Can you work these out from the model? Positions are in its coordinate system, mm. Face numbers are marked on the shaded views. A direction names the side the tool comes from. Round coordinates to 2 decimals unless told otherwise and drop trailing zeros. Loops run counter-clockwise (first coordinate to the right, second up) from the corner with the lowest first, then second, coordinate; pieces in that order, holes last. Notation, with made-up numbers: M -36.5,-20 L 5.5,-20 A11 cw 5.5,0 Z; hole C -33,4.5 d5. An arc over 180 degrees is marked long. Answer as CSV lines item,"result".
from build123d import *

# Parameters (mm, degrees)
SKETCH_1_W          = 50
SKETCH_1_H          = 25
EXTRUDE_1_DEPTH     = 2
SKETCH_2_W          = 15.416574513
SKETCH_2_H          = 15.10736158
EXTRUDE_2_DEPTH     = 16.5
SKETCH_2_6_W        = 4.64276656
SKETCH_2_6_H        = 12.070908618
SKETCH_2_6_W_2      = 4.657076635
SKETCH_2_6_H_2      = 15.10736158
EXTRUDE_3_DEPTH     = 8
SKETCH_3_R          = 1.5
CUT_EXTRUDE_1_DEPTH = 33.457664734
FILLET_1_R          = 2


with BuildPart() as part:
    # Sketch 1 → Extrude 1 (new body)
    with BuildSketch(Plane(origin=(0, 0, 0), x_dir=(1, 0, 0), z_dir=(0, 1, 0))):
        Rectangle(SKETCH_1_W, SKETCH_1_H)
    extrude(amount=EXTRUDE_1_DEPTH)

    # Sketch 2 → Extrude 2 (add)
    with BuildSketch(Plane(origin=(0, 2, 0), x_dir=(1, 0, 0), z_dir=(0, 1, 0))):
        with Locations((6.307789338, 0)):
            Rectangle(SKETCH_2_W, SKETCH_2_H)
    extrude(amount=EXTRUDE_2_DEPTH)

    # Sketch 2_6 → Extrude 3 (add)
    with BuildSketch(Plane(origin=(0, 2, 0), x_dir=(1, 0, 0), z_dir=(0, 1, 0))):
        with Locations((-21.10123104, 1.518226481)):
            Rectangle(SKETCH_2_6_W, SKETCH_2_6_H)
        with Locations((21.418251887, 0)):
            Rectangle(SKETCH_2_6_W_2, SKETCH_2_6_H_2)
    extrude(amount=EXTRUDE_3_DEPTH)

    # Sketch 3 → Cut-Extrude 1 (cut, through all)
    with BuildSketch(Plane(origin=(0, 2, 0), x_dir=(1, 0, 0), z_dir=(0, 1, 0))):
        with Locations(Location((-22.25, 10.25, 0), (0, 0, 270))):
            Circle(SKETCH_3_R)
        with Locations(Location((22.25, 10.25, 0), (0, 0, 90))):
            Circle(SKETCH_3_R)
        with Locations(Location((22.25, -10.25, 0), (0, 0, 270))):
            Circle(SKETCH_3_R)
        with Locations(Location((-22.25, -10.25, 0), (0, 0, 90))):
            Circle(SKETCH_3_R)
    extrude(amount=-CUT_EXTRUDE_1_DEPTH, mode=Mode.SUBTRACT)

    # Fillet 1
    fillet_1_edges = [part.edges().sort_by_distance(p)[0] for p in [
        (25, 1, 12.5),
        (-25, 1, 12.5),
        (-25, 1, -12.5),
        (25, 1, -12.5),
    ]]
    fillet(fillet_1_edges, radius=FILLET_1_R)


solid = part.part
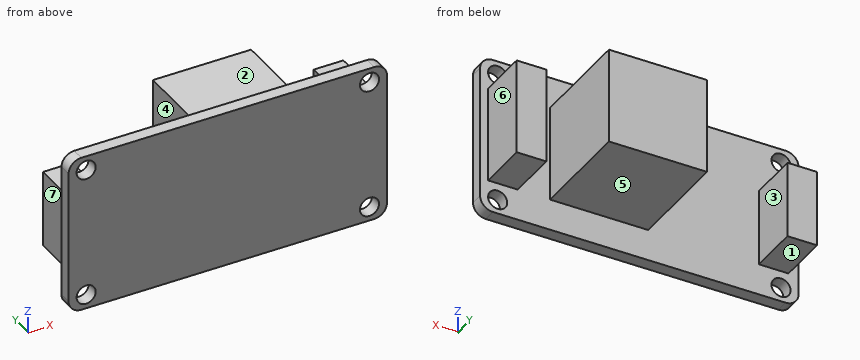
Item 1: If we section it at B-B on x = 22.25: Write out the boundary of the cut face in (y, z).
Output:
outline,"M 0,-12.5 L 2,-12.5 L 2,-11.75 L 0,-11.75 Z; M 0,-8.75 L 2,-8.75 L 2,-7.55 L 10,-7.55 L 10,7.55 L 2,7.55 L 2,8.75 L 0,8.75 Z; M 0,11.75 L 2,11.75 L 2,12.5 L 0,12.5 Z"
Item 2: If I drill on line 1 along X through (y, z) = (0.5, -10.25); line 2 along X through (y, z) = (8.25, -6.25); line 3 along X through (y, z) = (4.75, 5.5), over which ranges is the centre line in solid material (lowest first)? Write a range as from..to.
Output:
line 1,"x = -25..-23.75, -20.75..20.75, 23.75..25"
line 2,"x = -23.42..-18.78, -1.4..14.02, 19.09..23.75"
line 3,"x = -1.4..14.02, 19.09..23.75"
Item 3: If we section it at C-C on x = 0: Write out the boundary of the cut face in (y, z).
Output:
outline,"M 0,-12.5 L 2,-12.5 L 2,-7.55 L 18.5,-7.55 L 18.5,7.55 L 2,7.55 L 2,12.5 L 0,12.5 Z"
Item 4: We'd pull the mould along Z, two halves only. Please class the marked faces 1, 2 and 3: released by +Z, released by -Z, zero draft, split by the parting line, or undercut.
Output:
face 1,"released by -Z"
face 2,"released by +Z"
face 3,"zero draft"
Item 5: If we section it at D-D on x = -22.25: Write out the boundary of the cut face in (y, z), then the cut area to 3 significant figures.
Output:
outline,"M 0,-12.5 L 2,-12.5 L 2,-11.75 L 0,-11.75 Z; M 0,-8.75 L 2,-8.75 L 2,-7.55 L 10,-7.55 L 10,4.52 L 2,4.52 L 2,8.75 L 0,8.75 Z; M 0,11.75 L 2,11.75 L 2,12.5 L 0,12.5 Z"
area,"135 mm2"
Item 6: If we section it at A-A on y = 4.75: Write out the boundary of the cut face in (x, z).
Output:
outline,"M -23.42,-7.55 L -18.78,-7.55 L -18.78,4.52 L -23.42,4.52 Z; M -1.4,-7.55 L 14.02,-7.55 L 14.02,7.55 L -1.4,7.55 Z; M 19.09,-7.55 L 23.75,-7.55 L 23.75,7.55 L 19.09,7.55 Z"
Item 7: On a 3-axis mill with a long thin cutter (end or side, diameter ignored), from which of +Z, -Z, +X, -X, +Y, -Y can I reach the whole of each face in a straight line? I mean the marked faces 4, 5, 6 and 7. Say none if no direction works.
Output:
face 4,"+Z, -Z, +Y"
face 5,"-Z, +X, -X, +Y"
face 6,"+Z, -Z, +X, +Y"
face 7,"+Z, -Z, -X, +Y"
Item 8: Will these pins go through, and if not, where does the flat tip stop? pin 1 (5 mm diameter, centred on x = 12.5, y = 16.5, fed in from -Z); pin 2 (2.5 mm diameter, centred on x = -20, y = 7, fed in from +Z); pin 3 (3 mm diameter, centred on x = -7, z = 8, fed in from +Y).
Output:
pin 1,"stops at z = -7.55"
pin 2,"stops at z = 4.52"
pin 3,"stops at y = 2"
